Geometry check sheet. Reference: the model listing, model coordinates, mm. Give positions to 0.01 mm unless a question says otherwise; leave off trailing zeros. Loops run counter-clockwise (first coordinate to the right, second up) from the corner with the lowest first, then second, coordinate; pieces in that order, holes last. Notation, with made-up numbers: (42.25, 2) -> (87.25, 2) arc R20 cw to (87.25, 30) -> close; hole circle Ø7 at (73.5, 80). An arc over 180 degrees is marked (long way). Answer as a JSON object with one key per item and string values.
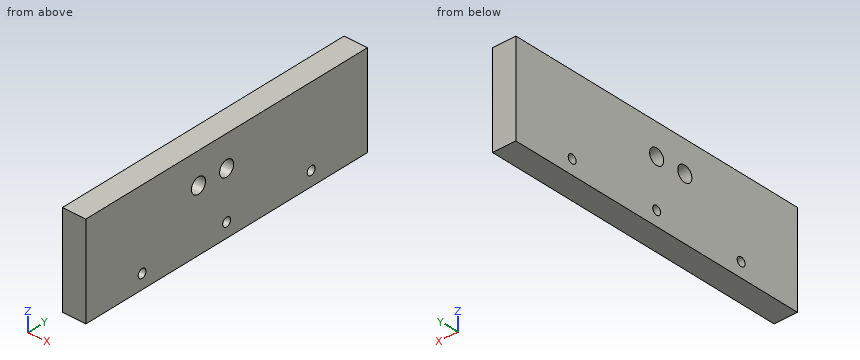
from build123d import *

# Parameters (mm, degrees)
SKETCH1_W           = 9.525
SKETCH1_H           = 127
BOSS_EXTRUDE1_DEPTH = 38.1
SKETCH2_R           = 1.778
CUT_EXTRUDE1_DEPTH  = 10.525
SKETCH3_R           = 3.175
CUT_EXTRUDE2_DEPTH  = 38.1


with BuildPart() as part:
    # Sketch1 → Boss-Extrude1 (new body)
    with BuildSketch(Plane.XY):
        with Locations((4.7625, 63.5)):
            Rectangle(SKETCH1_W, SKETCH1_H)
    extrude(amount=BOSS_EXTRUDE1_DEPTH)

    # Sketch2 → Cut-Extrude1 (cut, through all)
    with BuildSketch(Plane.ZY):
        with Locations((5.9182, 101.6)):
            Circle(SKETCH2_R)
        with Locations((5.9182, 63.5)):
            Circle(SKETCH2_R)
        with Locations((5.9182, 25.4)):
            Circle(SKETCH2_R)
    extrude(amount=-CUT_EXTRUDE1_DEPTH, mode=Mode.SUBTRACT)

    # Sketch3 → Cut-Extrude2 (cut)
    with BuildSketch(Plane(origin=(9.525, 0, 0), x_dir=(0, 0, -1), z_dir=(1, 0, 0))):
        with Locations((-25.4, 63.5)):
            Circle(SKETCH3_R)
        with Locations((-25.4, 50.8)):
            Circle(SKETCH3_R)
    extrude(amount=-CUT_EXTRUDE2_DEPTH, mode=Mode.SUBTRACT)


solid = part.part
1) Section check B-B on z = 25.4. Record the cut outline in (x, y) (3 decimals), plus the area to 3 significant figures.
Geometry check:
{"outline": "(0, 0) -> (9.525, 0) -> (9.525, 47.625) -> (0, 47.625) -> close; (0, 53.975) -> (9.525, 53.975) -> (9.525, 60.325) -> (0, 60.325) -> close; (0, 66.675) -> (9.525, 66.675) -> (9.525, 127) -> (0, 127) -> close", "area": "1,090 mm2"}
2) Section check D-D on y = 63.5. Record the cut outline in (x, z) (3 decimals).
Geometry check:
{"outline": "(0, 0) -> (9.525, 0) -> (9.525, 4.14) -> (0, 4.14) -> close; (0, 7.696) -> (9.525, 7.696) -> (9.525, 22.225) -> (0, 22.225) -> close; (0, 28.575) -> (9.525, 28.575) -> (9.525, 38.1) -> (0, 38.1) -> close"}
3) Section check C-C on x = 4.25. Record the cut outline in (y, z) (3 decimals), plus the area to 3 significant figures.
Geometry check:
{"outline": "(0, 0) -> (127, 0) -> (127, 38.1) -> (0, 38.1) -> close; hole circle Ø3.556 at (25.4, 5.918); hole circle Ø6.35 at (50.8, 25.4); hole circle Ø6.35 at (63.5, 25.4); hole circle Ø3.556 at (63.5, 5.918); hole circle Ø3.556 at (101.6, 5.918)", "area": "4,750 mm2"}
4) Material ranges on line 1 along Y through (x, z) = (7.5, 25); line 2 along Y through (x, z) = (5, 25.4) (3 decimals); line 3 along Z through (x, y) = (7.25, 101.6), recorded low to high. Write a range as from..to.
Geometry check:
{"line 1": "y = 0..47.65, 53.95..60.35, 66.65..127", "line 2": "y = 0..47.625, 53.975..60.325, 66.675..127", "line 3": "z = 0..4.14, 7.7..38.1"}
5) Section check A-A on y = 25.4. Record the cut outline in (x, z) (3 decimals), plus the area to 3 significant figures.
Geometry check:
{"outline": "(0, 0) -> (9.525, 0) -> (9.525, 4.14) -> (0, 4.14) -> close; (0, 7.696) -> (9.525, 7.696) -> (9.525, 38.1) -> (0, 38.1) -> close", "area": "329 mm2"}
